Autodesk Inventor part; units mm, degrees
ref_plane "YZ Plane" through (0, 0, 0) normal (1, 0, 0) x (0, 1, 0)
ref_plane "XZ Plane" through (0, 0, 0) normal (0, 1, 0) x (-1, 0, 0)
ref_plane "XY Plane" through (0, 0, 0) normal (0, 0, 1) x (1, 0, 0)
sketch "Boceto1" plane through (0, 0, 0) normal (0, 0, 1) x (1, 0, 0)
  line L0 (-13.125, -37.65) -> (13.125, -37.65)
  line L1 (13.125, -37.65) -> (13.125, 37.65)
  line L2 (13.125, 37.65) -> (-13.125, 37.65)
  line L3 (-13.125, 37.65) -> (-13.125, -37.65)
  line L4 (-13.125, -37.65) -> (13.125, 37.65) construction
  line L5 (13.125, -37.65) -> (-13.125, 37.65) construction
  line L6 (0, -37.65) -> (0, -35.15)
  line L7 (0, -35.15) -> (10.5, -35.15)
  line L8 (10.5, -35.15) -> (-10.5, -35.15)
  circle A0 centre (10.5, -35.15) radius 1.5
  circle A1 centre (-10.5, -35.15) radius 1.5
  line L9 (-10.5, -35.15) -> (-10.5, 2.15)
  circle A2 centre (-10.5, 2.15) radius 1.5
  point P0 (0, 0)
  dimension "d0" = 26.25
  dimension "d1" = 75.3
  dimension "d2" = 2.5
  dimension "d3" = 10.5
  dimension "d4" = 21
  dimension "d5" = 3
  dimension "d6" = 3
  dimension "d7" = 37.3
  dimension "d8" = 3
extrude "Extrusión1" add sketch "Boceto1" along normal blind 1.6
sketch "Boceto3" plane through (0, 0, 0) normal (0, 0, -1) x (-1, 0, 0)
  line L0 (-13.125, 37.65) -> (13.125, 37.65)
  line L1 (8.7698, 11.9975) -> (-8.7698, 11.9975)
  line L2 (-8.7698, 11.9975) -> (-8.7698, 37.65)
  line L3 (-8.7698, 37.65) -> (8.7698, 37.65)
  line L4 (8.7698, 37.65) -> (8.7698, 11.9975)
  line L5 (8.7698, 11.9975) -> (-8.7698, 37.65) construction
  line L6 (-8.7698, 11.9975) -> (8.7698, 37.65) construction
  line L7 (7.9072, -18.1146) -> (-7.9072, -18.1146)
  line L8 (-7.9072, -18.1146) -> (-7.9072, -2.2044)
  line L9 (-7.9072, -2.2044) -> (7.9072, -2.2044)
  line L10 (7.9072, -2.2044) -> (7.9072, -18.1146)
  line L11 (7.9072, -18.1146) -> (-7.9072, -2.2044) construction
  line L12 (-7.9072, -18.1146) -> (7.9072, -2.2044) construction
  point P0 (0, 0)
  point P1 (0, 24.8238)
  point P2 (0, -10.1595)
extrude "Extrusión2" add sketch "Boceto3" along normal blind 1.6
sketch "Boceto4" plane through (0, 0, -1.6) normal (0, 0, -1) x (-1, 0, 0)
  line L0 (8.003, 29.9035) -> (-8.003, 29.9035)
  line L1 (-8.003, 29.9035) -> (-8.003, 12.6515)
  line L2 (-8.003, 12.6515) -> (8.003, 12.6515)
  line L3 (8.003, 12.6515) -> (8.003, 29.9035)
  line L4 (8.003, 29.9035) -> (-8.003, 12.6515) construction
  line L5 (-8.003, 29.9035) -> (8.003, 12.6515) construction
  point P0 (0, 0)
  point P1 (0, 21.2775)
extrude "Extrusión3" add sketch "Boceto4" along normal blind 2.5
sketch "Boceto5" plane through (-13.125, 37.65, 1.6) normal (0, 1, 0) x (1, 0, 0)
  line L0 (21.8948, 3.2) -> (4.3552, 3.2)
  line L1 (21.8948, 1.6) -> (21.8948, 3.2)
  line L2 (4.3552, 3.2) -> (21.8948, 3.2)
  line L3 (21.8948, 3.2) -> (21.8948, 1.6)
  line L4 (21.8948, 1.6) -> (4.3552, 1.6)
  line L5 (4.3552, 1.6) -> (4.3552, 3.2)
  point P0 (13.125, 1.6)
extrude "Extrusión4" cut sketch "Boceto5" against normal blind 0.1
sketch "Boceto6" plane through (0, 0, -1.6) normal (0, 0, -1) x (-1, 0, 0)
  line L0 (5.9327, -11.7926) -> (-0.4732, -11.7926)
  line L1 (-0.4732, -11.7926) -> (-0.4732, -6.1147)
  line L2 (-0.4732, -6.1147) -> (5.9327, -6.1147)
  line L3 (5.9327, -6.1147) -> (5.9327, -11.7926)
  line L4 (5.9327, -11.7926) -> (-0.4732, -6.1147) construction
  line L5 (-0.4732, -11.7926) -> (5.9327, -6.1147) construction
  point P0 (0, 0)
  point P1 (2.7298, -8.9537)
extrude "Extrusión5" add sketch "Boceto6" along normal blind 1
sketch "Boceto7" plane through (0, 0, 0) normal (0, 0, -1) x (-1, 0, 0)
  line L0 (13.125, 37.65) -> (13.125, -37.65)
  line L1 (13.125, -32.0293) -> (6.4423, -32.0293)
  line L2 (6.4423, -32.0293) -> (6.4423, -25.9874)
  line L3 (6.4423, -25.9874) -> (13.125, -25.9874)
  line L4 (13.125, -25.9874) -> (13.125, -32.0293)
  point P0 (0, 0)
extrude "Extrusión6" add sketch "Boceto7" along normal blind 5.5
sketch "Boceto8" plane through (0, 0, 0) normal (0, 0, -1) x (-1, 0, 0)
  line L0 (13.125, 37.65) -> (13.125, -37.65)
  line L1 (13.125, -25.3323) -> (9.5724, -25.3323)
  line L2 (9.5724, -25.3323) -> (9.5724, -19.5088)
  line L3 (9.5724, -19.5088) -> (13.125, -19.5088)
  line L4 (13.125, -19.5088) -> (13.125, -25.3323)
  line L5 (13.125, -37.65) -> (-13.125, -37.65)
  line L6 (-1.4923, -37.65) -> (-7.8981, -37.65)
  line L7 (-7.8981, -37.65) -> (-7.8981, -33.558)
  line L8 (-7.8981, -33.558) -> (-1.4923, -33.558)
  line L9 (-1.4923, -33.558) -> (-1.4923, -37.65)
  line L10 (-6.5151, -30.4279) -> (-11.3195, -30.4279)
  line L11 (-11.3195, -30.4279) -> (-11.3195, -25.3323)
  line L12 (-11.3195, -25.3323) -> (-6.5151, -25.3323)
  line L13 (-6.5151, -25.3323) -> (-6.5151, -30.4279)
  point P0 (0, 0)
extrude "Extrusión7" add sketch "Boceto8" along normal blind 3
sketch "Boceto9" plane through (-13.125, -37.65, 1.6) normal (0, -1, 0) x (1, 0, 0)
  line L0 (14.6173, -4.6) -> (21.0231, -4.6)
  line L1 (21.0231, -1.6) -> (21.0231, -4.6)
  line L2 (14.6173, -4.6) -> (21.0231, -4.6)
  line L3 (21.0231, -4.6) -> (21.0231, -1.6)
  line L4 (21.0231, -1.6) -> (14.6173, -1.6)
  line L5 (14.6173, -1.6) -> (14.6173, -4.6)
  point P0 (13.125, -1.6)
extrude "Extrusión8" cut sketch "Boceto9" against normal blind 0.1
sketch "Boceto10" plane through (-13.125, -37.65, 1.6) normal (-1, 0, 0) x (0, 0, 1)
  line L0 (-4.6, 12.3177) -> (-4.6, 18.1412)
  line L1 (-1.6, 12.3177) -> (-1.6, 11.6626)
  line L2 (-4.6, 18.1412) -> (-1.6, 18.1412)
  line L3 (-1.6, 18.1412) -> (-1.6, 12.3177)
  line L4 (-1.6, 12.3177) -> (-4.6, 12.3177)
  line L5 (-4.6, 12.3177) -> (-4.6, 18.1412)
  line L6 (-7.1, 5.6207) -> (-7.1, 11.6626)
  line L7 (-1.6, 5.6207) -> (-7.1, 5.6207)
  line L8 (-7.1, 11.6626) -> (-1.6, 11.6626)
  line L9 (-1.6, 11.6626) -> (-1.6, 5.6207)
  line L10 (-1.6, 5.6207) -> (-7.1, 5.6207)
  line L11 (-7.1, 5.6207) -> (-7.1, 11.6626)
  point P0 (-1.6, 37.65)
extrude "Extrusión9" cut sketch "Boceto10" against normal blind 0.1
properties part number "ESP32"
Verification items for the finished model (mm, model axes). A direction names the side the tool comes from. Give positions to 0.01 mm unless a question says otherwise; leave off trailing zeros. Write each loop counter-clockwise with the first axis right and the second up, starting at its lowest first coordinate (ties: lowest second). Pieces come first, ordered by that corner, then holes. Notation, with made-up numbers: M 79.25,81 L 118.25,81 A7 ccw 118.25,90 Z; hole C -21,58.5 d4. An arc over 180 degrees is marked long. Write item = value, one per line.
(1) Go/stop test with flat-tipped pins: pin 1 Ø3 at (x, z) = (-8.5, -4) entering from -Y; pin 2 Ø1.1 at (x, z) = (-2, -2) entering from +Y; pin 3 Ø12 at (x, y) = (9.5, 26.5) entering from -Z. Record where each tip stops, or that it passes through.
Found:
pin_1 = -32.03
pin_2 = 37.55
pin_3 = -4.1
(2) Draft check along X on faces 1 (the face through (5, -37.55, -1)), 2 (the face through (10.175, -33.686, 0.789)), 3 (the face through (6.515, -28, -1)), 4 (the face through (8.003, 21, -3)). Enter one of: released by +X, released by -X, zero draft, split by the parting line, or undercut.
Found:
face_1 = zero draft
face_2 = undercut
face_3 = undercut
face_4 = released by +X
(3) Sectioned sample at B-B (y = -35.15). Record the cut outline in (x, z) (3 decimals).
Found:
outline = M -13.125,0 L -12,0 L -12,1.6 L -13.125,1.6 Z; M -9,0 L 1.492,0 L 1.492,-3 L 7.898,-3 L 7.898,0 L 9,0 L 9,1.6 L -9,1.6 Z; M 12,0 L 13.125,0 L 13.125,1.6 L 12,1.6 Z
(4) Access from +Z, -Z, +X, -X, +Y, -Y to the whole of each face (thin tool, end or side, straight path). Record for faces 5 (the face through (5, -33.558, -1)), 6 (the face through (9, -30.428, -1)), 7 (the face through (0, 37.55, -1)), 8 (the face through (7.898, -36, -1)), 9 (the face through (-13.025, -22, -2)).
Found:
face_5 = -Z, +X, -X
face_6 = -Z, +X
face_7 = -Z, +X, -X, +Y
face_8 = -Z, +X, -Y
face_9 = -Z, -X, +Y, -Y
(5) Sectioned sample at A-A (x = -10.5). Record the cut outline in (y, z), then the cut area to 3 significant figures.
Found:
outline = M -37.65,0 L -36.65,0 L -36.65,1.6 L -37.65,1.6 Z; M -33.65,0 L -32.03,0 L -32.03,-5.5 L -25.99,-5.5 L -25.99,0 L -25.33,0 L -25.33,-3 L -19.51,-3 L -19.51,0 L 0.65,0 L 0.65,1.6 L -33.65,1.6 Z; M 3.65,0 L 37.65,0 L 37.65,1.6 L 3.65,1.6 Z
area = 162 mm2
(6) Sectioned sample at D-D (y = 2.15). Record the cut outline in (x, z) (3 decimals), then the cut area to 3 significant figures.
Found:
outline = M -13.125,0 L -12,0 L -12,1.6 L -13.125,1.6 Z; M -9,0 L 13.125,0 L 13.125,1.6 L -9,1.6 Z
area = 37.2 mm2
(7) Material ranges on line 1 (Y direction, x = -10.5, z = 0.6); line 2 (X direction, y = -35.15, z = 0.7) (3 decimals); line 3 (Y direction, x = -9.75, z = -1.5), recorded low to high.
Found:
line_1 = -37.65 to -36.65, -33.65 to 0.65, 3.65 to 37.65
line_2 = -13.125 to -12, -9 to 9, 12 to 13.125
line_3 = -32.03 to -25.99, -25.33 to -19.51
(8) Sectioned sample at C-C (x = 10.5). Record the cut outline in (y, z), then the cut area to 3 significant figures.
Found:
outline = M -37.65,0 L -36.65,0 L -36.65,1.6 L -37.65,1.6 Z; M -33.65,0 L -30.43,0 L -30.43,-3 L -25.33,-3 L -25.33,0 L 37.65,0 L 37.65,1.6 L -33.65,1.6 Z
area = 131 mm2
